Source: CAD feature listing. Evaluate the final solid. Frame: model axes, mm. A direction names the side the tool comes from. Round coordinates to 2 decimals unless told otherwise and drop trailing zeros. Order: outer loops, then holes, each group sorted by start corner. A loop starts at its lowest first (then second) coordinate and runs counter-clockwise, first axis right, second up. Notation, with made-up numbers: (18.25, 70.25) - (50.25, 70.25) arc R16 ccw to (50.25, 81.25) - close; hole circle Ø3 at (-21, -28.75). An arc over 180 degrees is marked (long way). Use one line per item in the form item = value. Start each with the question number.
Q1. Cut plane A-A, the plane x = 0. Return the cut outline in (y, z) (3 decimals).
Q2. Draft query along X for faces 4 (the flat face through (7, -7, 12.7)), 5 (the cylindrical face through (28.547, 1.256, -3.131)), 6 (the cylindrical face through (7.133, -4.155, 3.308)). Return one class per face: released by +X, released by -X, zero draft, split by the parting line, or undercut.
Q3. Set-up query: faces 1 (the flat face through (-6, -6, -6.35)), 2 (the flat face through (-2.756, -8.837, 3.308)), 3 (the flat face through (-12, -12, 0)). Return all of +Z, -Z, +X, -X, +Y, -Y with unobstructed straight access to the full face (end or side cutting, diameter ignored); none if empty.
Q4. Ray query, line 1 (Y direction, x = -13, z = -1); line 2 (X direction, y = 21, z = -2.5); line 3 (Z direction, x = 23, y = -4). Return the intervals inside material, ascending. Write a range as [from, to].
Q5. Cut plane C-C, the plane y = 0. Give the number of separate pieces and of enclosed holes in the cut face, and give its area (3 significant figures).
Q6. Pin query (flat end, axial travel): pin 1 Ø0.6 at (x, z) = (-9.5, 4) entering from +Y; pin 2 Ø8 at (x, y) = (-22, -5.5) entering from +Z; pin 3 Ø3 at (x, z) = (1, -2.5) entering from +Y (3 decimals); pin 4 Ø4 at (x, y) = (11.91, -20.62) entering from -Z. Return the tip coordinate at first contact, or that it passes through.
Q7. Cut plane B-B, the plane z = 9.5. Return the cut outline in (x, y) (3 decimals), and give its area (3 significant figures).
from build123d import *

# Parameters (mm, degrees)
SKETCH1_R           = 15.875
BOSS_EXTRUDE1_DEPTH = 12.7
SKETCH4_R           = 28.575
BOSS_EXTRUDE3_DEPTH = 6.35
CUT_EXTRUDE2_DEPTH  = 19.05
SKETCH6_R           = 2.54
CUT_EXTRUDE3_DEPTH  = 6.35


with BuildPart() as part:
    # Sketch1 → Boss-Extrude1 (new body)
    with BuildSketch(Plane.XY):
        Circle(SKETCH1_R)
    extrude(amount=BOSS_EXTRUDE1_DEPTH)

    # Sketch4 → Boss-Extrude3 (add)
    with BuildSketch(Plane(origin=(0, 0, 0), x_dir=(-1, 0, 0), z_dir=(0, 0, -1))):
        Circle(SKETCH4_R)
    extrude(amount=BOSS_EXTRUDE3_DEPTH)

    # Sketch5 → Cut-Extrude2 (cut)
    with BuildSketch(Plane.XY.offset(12.7)):
        with BuildLine():
            Line((6.77626362, -7.672832876), (5.76026362, -5.913069256))
            ThreePointArc((5.76026362, -5.913069256), (7.149039708, -4.1275), (8.001, -2.032))
            Line((8.001, -2.032), (10.033, -2.032))
            Line((10.033, -2.032), (10.033, 2.032))
            Line((10.033, 2.032), (8.001, 2.032))
            ThreePointArc((8.001, 2.032), (7.149039708, 4.1275), (5.76026362, 5.913069256))
            Line((5.76026362, 5.913069256), (6.77626362, 7.672832876))
            Line((6.77626362, 7.672832876), (3.25673638, 9.704832876))
            Line((3.25673638, 9.704832876), (2.24073638, 7.945069256))
            ThreePointArc((2.24073638, 7.945069256), (0, 8.255), (-2.24073638, 7.945069256))
            Line((-2.24073638, 7.945069256), (-3.25673638, 9.704832876))
            Line((-3.25673638, 9.704832876), (-6.77626362, 7.672832876))
            Line((-6.77626362, 7.672832876), (-5.76026362, 5.913069256))
            ThreePointArc((-5.76026362, 5.913069256), (-7.149039708, 4.1275), (-8.001, 2.032))
            Line((-8.001, 2.032), (-10.033, 2.032))
            Line((-10.033, 2.032), (-10.033, -2.032))
            Line((-10.033, -2.032), (-8.001, -2.032))
            ThreePointArc((-8.001, -2.032), (-7.149039708, -4.1275), (-5.76026362, -5.913069256))
            Line((-5.76026362, -5.913069256), (-6.77626362, -7.672832876))
            Line((-6.77626362, -7.672832876), (-3.25673638, -9.704832876))
            Line((-3.25673638, -9.704832876), (-2.24073638, -7.945069256))
            ThreePointArc((-2.24073638, -7.945069256), (0, -8.255), (2.24073638, -7.945069256))
            Line((2.24073638, -7.945069256), (3.25673638, -9.704832876))
            Line((3.25673638, -9.704832876), (6.77626362, -7.672832876))
        make_face()
    extrude(amount=-CUT_EXTRUDE2_DEPTH, mode=Mode.SUBTRACT)

    # Sketch6 → Cut-Extrude3 (cut)
    with BuildSketch(Plane(origin=(0, 0, -6.35), x_dir=(-1, 0, 0), z_dir=(0, 0, -1))):
        with Locations((-23.8125, 0)):
            Circle(SKETCH6_R)
        with Locations((-11.90625, 20.622229928)):
            Circle(SKETCH6_R)
        with Locations((11.90625, 20.622229928)):
            Circle(SKETCH6_R)
        with Locations((23.8125, 0)):
            Circle(SKETCH6_R)
        with Locations((11.90625, -20.622229928)):
            Circle(SKETCH6_R)
        with Locations((-11.90625, -20.622229928)):
            Circle(SKETCH6_R)
    extrude(amount=-CUT_EXTRUDE3_DEPTH, mode=Mode.SUBTRACT)


solid = part.part
Completed:
q1.outline = (-28.575, -6.35) - (-8.255, -6.35) - (-8.255, 12.7) - (-15.875, 12.7) - (-15.875, 0) - (-28.575, 0) - close; (8.255, -6.35) - (28.575, -6.35) - (28.575, 0) - (15.875, 0) - (15.875, 12.7) - (8.255, 12.7) - close
q2.face_4 = zero draft
q2.face_5 = split by the parting line
q2.face_6 = undercut
q3.face_1 = -Z, +X, -X, +Y, -Y
q3.face_2 = +Z, -Z
q3.face_3 = +Z
q4.line_1 = [-25.45, -22.91], [-18.33, 18.33], [22.91, 25.45]
q4.line_2 = [-19.38, -14.42], [-9.39, 9.39], [14.42, 19.38]
q4.line_3 = [-6.35, 0]
q5.separate_pieces = 4
q5.enclosed_holes = 0
q5.area = 319 mm2
q6.pin_1 = 12.94
q6.pin_2 = 0
q6.pin_3 = 28.575
q6.pin_4 = through
q7.outline = circle Ø31.75 at (0, 0); hole (-10.033, -2.032) - (-8.001, -2.032) arc R8.255 ccw to (-5.76, -5.913) - (-6.776, -7.673) - (-3.257, -9.705) - (-2.241, -7.945) arc R8.255 ccw to (2.241, -7.945) - (3.257, -9.705) - (6.776, -7.673) - (5.76, -5.913) arc R8.255 ccw to (8.001, -2.032) - (10.033, -2.032) - (10.033, 2.032) - (8.001, 2.032) arc R8.255 ccw to (5.76, 5.913) - (6.776, 7.673) - (3.257, 9.705) - (2.241, 7.945) arc R8.255 ccw to (-2.241, 7.945) - (-3.257, 9.705) - (-6.776, 7.673) - (-5.76, 5.913) arc R8.255 ccw to (-8.001, 2.032) - (-10.033, 2.032) - close
q7.area = 532 mm2
